Geometry check sheet. Reference: the model listing, model coordinates, mm. A direction names the side the tool comes from. Coordinates: 2 decimals unless noted, no trailing zeros. Order: outer loops, then holes, each group sorted by start corner. A loop starts at its lowest first (then second) coordinate and runs counter-clockwise, first axis right, second up. Notation, with made-up numbers: M 77.5,10 L 104.5,10 A33 ccw 104.5,42 Z; hole C -10.5,57 d6. An arc over 180 degrees is marked long. One line per item, written item: value. Start each with the question number.
1) Sectioned sample at C-C, the plane x = -2.25. Enter the section's corners in (y, z).
2) Sectioned sample at A-A, the plane x = 6. Enter the section's corners in (y, z).
3) Draft check along Z on faces 1 (the cylindrical face through (8.86, 0.11, -2.54)), 2 (the flat face through (4, -7, 45)), 3 (the flat face through (4, -7, -5)), 4 (the flat face through (4, -5.5, 0)). Enter one of: pulls with the +Z half, pulls with the -Z half, needs draft (parallel to the pull), parting line crosses it, or undercut.
4) Thickness scan on L1, parallel to Z at x = 5.5, y = -7.75; L2, parallel to Y at x = 7.25, z = -2; L3, parallel to X at y = 7.5, z = 35. Record the ranges inside material, lowest first. Write a range as from..to.
5) Go/stop test with flat-tipped pins: P1, Ø0.8, axis at x = 16.5, z = 18, coming from the -Y side; P2, Ø16, axis at x = 3.86, y = -0.11, coming from the +Z side; P3, Ø3, axis at x = 6, z = 37.5, coming from the +Y side; P4, Ø1, axis at y = -9, z = 7, coming from the +X side. Record where each tip stops, or that it passes through.
6) Access from +Z, -Z, +X, -X, +Y, -Y to the whole of each face (thin tool, end or side, straight path). Record for faces 5 (the flat face through (17, 0, 28)), 6 (the flat face through (3.7, -5.5, 40)), 7 (the cylindrical face through (8.86, 0.11, 42.46)).
7) Sectioned sample at D-D, the plane y = 8.5. Enter the section's corners in (x, z), then the cut area to 3 significant figures.
8) Sectioned sample at B-B, the plane y = -1. Enter the section's corners in (x, z).
```python
from build123d import *

# Parameters (mm, degrees)
SKETCH1_R           = 15
SKETCH1_R_2         = 12.5
BOSS_EXTRUDE1_DEPTH = 40
SKETCH2_R           = 15
BOSS_EXTRUDE2_DEPTH = 5
SKETCH3_R           = 15
BOSS_EXTRUDE3_DEPTH = 5
SKETCH4_R           = 5
BOSS_EXTRUDE4_DEPTH = 160
SKETCH5_W           = 16
SKETCH5_H           = 12
CUT_EXTRUDE1_DEPTH  = 160


with BuildPart() as part:
    # Sketch1 → Boss-Extrude1 (new body)
    with BuildSketch(Plane.XY):
        with Locations((3.864023938, -0.112000694)):
            Circle(SKETCH1_R)
        with Locations((3.864023938, -0.112000694)):
            Circle(SKETCH1_R_2, mode=Mode.SUBTRACT)
    extrude(amount=BOSS_EXTRUDE1_DEPTH)

    # Sketch2 → Boss-Extrude2 (add)
    with BuildSketch(Plane.XY.offset(40)):
        with Locations((3.864023938, -0.112000694)):
            Circle(SKETCH2_R)
    extrude(amount=BOSS_EXTRUDE2_DEPTH)

    # Sketch3 → Boss-Extrude3 (add)
    with BuildSketch(Plane(origin=(0, 0, 0), x_dir=(-1, 0, 0), z_dir=(0, 0, -1))):
        with Locations((-3.864023938, -0.112000694)):
            Circle(SKETCH3_R)
    extrude(amount=BOSS_EXTRUDE3_DEPTH)


with BuildPart() as body_2:
    # Sketch4 → Boss-Extrude4 (new body)
    with BuildSketch(Plane(origin=(0, 0, -5), x_dir=(-1, 0, 0), z_dir=(0, 0, -1))):
        with Locations((-3.864023938, -0.112000694)):
            Circle(SKETCH4_R)
    extrude(amount=-BOSS_EXTRUDE4_DEPTH)


with BuildPart() as part_1:
    add(part.part)

    # Combine1: cut body 2
    add(body_2.part, mode=Mode.SUBTRACT)

    # Sketch5 → Cut-Extrude1 (cut)
    with BuildSketch(Plane(origin=(0, 0, 0), x_dir=(0, 0, -1), z_dir=(1, 0, 0))):
        with Locations((-20, -0.112000694)):
            Rectangle(SKETCH5_W, SKETCH5_H)
    extrude(amount=CUT_EXTRUDE1_DEPTH, mode=Mode.SUBTRACT)


solid = part_1.part
```
Final values:
1. outline: M -13.81,-5 L 13.59,-5 L 13.59,45 L -13.81,45 Z; hole M -11.01,0 L 10.79,0 L 10.79,40 L -11.01,40 Z
2. outline: M -14.96,-5 L -4.63,-5 L -4.63,0 L -12.43,0 L -12.43,40 L -4.63,40 L -4.63,45 L -14.96,45 Z; M 4.41,-5 L 14.74,-5 L 14.74,45 L 4.41,45 L 4.41,40 L 12.2,40 L 12.2,0 L 4.41,0 Z
3. face 1: needs draft
3. face 2: pulls with the +Z half
3. face 3: pulls with the -Z half
3. face 4: undercut
4. L1: z = -5..0, 40..45
4. L2: y = -14.72..-3.79, 3.57..14.5
4. L3: x = -9.06..-6.05, 13.78..16.79
5. P1: stops at y = -8.79
5. P2: stops at z = 45
5. P3: stops at y = 14.87
5. P4: stops at x = 16.3
6. face 5: +X
6. face 6: none
6. face 7: +Z, -Z
7. outline: M -8.42,-5 L 16.15,-5 L 16.15,45 L -8.42,45 Z; hole M -5.2,0 L 12.92,0 L 12.92,40 L -5.2,40 Z
7. area: 503 mm^2
8. outline: M -11.11,-5 L -1.06,-5 L -1.06,0 L -8.6,0 L -8.6,40 L -1.06,40 L -1.06,45 L -11.11,45 Z; M 8.78,-5 L 18.84,-5 L 18.84,12 L 16.33,12 L 16.33,0 L 8.78,0 Z; M 8.78,40 L 16.33,40 L 16.33,28 L 18.84,28 L 18.84,45 L 8.78,45 Z
